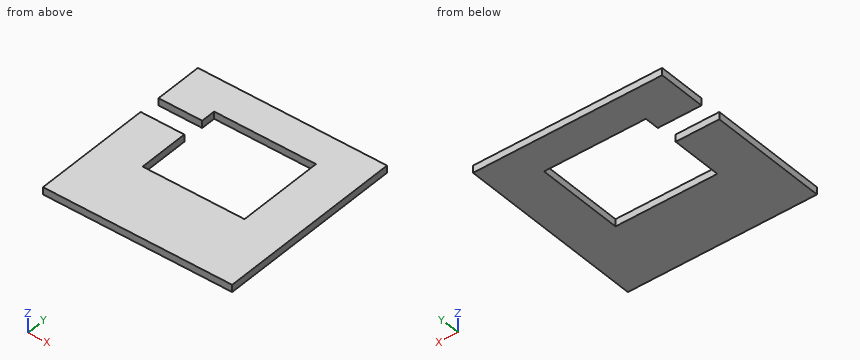
from build123d import *

# Parameters (mm, degrees)
SCHIZZO1_W                   = 130
SCHIZZO1_H                   = 130
ESTRUSIONE_ESTRUSIONE1_DEPTH = 5
SCHIZZO2_W                   = 70
SCHIZZO2_H                   = 60
TAGLIO_ESTRUSIONE1_DEPTH     = 5
SCHIZZO3_W                   = 30
SCHIZZO3_H                   = 15
TAGLIO_ESTRUSIONE2_DEPTH     = 10


with BuildPart() as part:
    # Schizzo1 → Estrusione-Estrusione1 (new body)
    with BuildSketch(Plane.XY):
        Rectangle(SCHIZZO1_W, SCHIZZO1_H)
    extrude(amount=ESTRUSIONE_ESTRUSIONE1_DEPTH)

    # Schizzo2 → Taglio-Estrusione1 (cut)
    with BuildSketch(Plane.XY.offset(5)):
        with Locations((0, 12)):
            Rectangle(SCHIZZO2_W, SCHIZZO2_H)
    extrude(amount=-TAGLIO_ESTRUSIONE1_DEPTH, mode=Mode.SUBTRACT)

    # Schizzo3 → Taglio-Estrusione2 (cut)
    with BuildSketch(Plane.XY.offset(5)):
        with Locations((-50, 24.5)):
            Rectangle(SCHIZZO3_W, SCHIZZO3_H)
    extrude(amount=-TAGLIO_ESTRUSIONE2_DEPTH, mode=Mode.SUBTRACT)


solid = part.part
Part model, mm, in its own coordinate system. Coordinates: 2 decimals unless noted, no trailing zeros. Write each loop counter-clockwise with the first axis right and the second up, starting at its lowest first coordinate (ties: lowest second). Pieces come first, ordered by that corner, then holes. Notation, with made-up numbers: M -35,2.5 L 20,2.5 A17 cw 20,27.5 Z; hole C 51.25,36.5 d6. An arc over 180 degrees is marked long. Return JSON: item names as keys, results as strings.
1. Saw through at C-C, the plane z = 1.7. Write the cut outline in (x, y).
Determined:
{"outline": "M -65,-65 L 65,-65 L 65,65 L -65,65 L -65,32 L -35,32 L -35,42 L 35,42 L 35,-18 L -35,-18 L -35,17 L -65,17 Z"}
2. Saw through at A-A, the plane y = -12.5. Write the cut outline in (x, z), then the cut area to 3 significant figures.
Determined:
{"outline": "M -65,0 L -35,0 L -35,5 L -65,5 Z; M 35,0 L 65,0 L 65,5 L 35,5 Z", "area": "300 mm²"}
3. Saw through at B-B, the plane x = -40. Write the cut outline in (y, z), then the cut area to 3 significant figures.
Determined:
{"outline": "M -65,0 L 17,0 L 17,5 L -65,5 Z; M 32,0 L 65,0 L 65,5 L 32,5 Z", "area": "575 mm²"}
4. Probe L1, parallel to Y at x = -4.5, z = 4.05; L2, parallel to X at y = 34, z = 3.2; L3, parallel to Y at x = -57, z = 3.5. List the from-to ranges inside material, lowest first.
Determined:
{"L1": "-65 to -18, 42 to 65", "L2": "-65 to -35, 35 to 65", "L3": "-65 to 17, 32 to 65"}
5. Flat gauge pins, fed straight in: pin 1 Ø12 at (x, y) = (-32, 35) entering from +Z; pin 2 Ø10 at (x, y) = (-28.5, -1) entering from -Z. Where does each tip first touch, or does it go through?
Determined:
{"pin 1": "z = 5", "pin 2": "through"}
